Could you check a few things on this model? Use its own coordinates, in mm. A direction names the side the tool comes from. Coordinates: 2 decimals unless noted, no trailing zeros. Loops run counter-clockwise (first coordinate to the right, second up) from the corner with the lowest first, then second, coordinate; pieces in that order, holes last. Notation, with made-up numbers: M 40,84 L 44,84 A30 cw 44,114 Z; hole C -29.75,-31.75 d8. An arc over 180 degrees is marked long. Write each question's results on one line, items separated by ' | '.
```python
from build123d import *

# Parameters (mm, degrees)
F0_R     = 12.5
F0_R_2   = 7
F1_DEPTH = 40
F2_DEPTH = 15


with BuildPart() as f1:
    # F0 (on Top) → F1 (new body)
    with BuildSketch(Plane.XY):
        Circle(F0_R)
        Circle(F0_R_2, mode=Mode.SUBTRACT)
    extrude(amount=F1_DEPTH)

    # F0 (on Top) → F2 (join)
    with BuildSketch(Plane.XY):
        Circle(F0_R_2)
        with BuildLine():
            ThreePointArc((1.658312, 2.5), (2.643382, 1.418637), (3, 0))
            ThreePointArc((3, 0), (-1.418637, -2.643382), (-1.658312, 2.5))
            ThreePointArc((-1.658312, 2.5), (0, 3), (1.658312, 2.5))
        make_face(mode=Mode.SUBTRACT)
        with BuildLine():
            Line((-1.658312, 2.5), (1.658312, 2.5))
            ThreePointArc((1.658312, 2.5), (0, 3), (-1.658312, 2.5))
        make_face()
    extrude(amount=F2_DEPTH)


solid = f1.part
```
(1) Imagine slicing it at C-C, the plane y = 4. List the corners of the cut face in (x, z) for me, and give its area (3 significant figures).
Reported:
outline: M -11.84,0 L 11.84,0 L 11.84,40 L 5.74,40 L 5.74,15 L -5.74,15 L -5.74,40 L -11.84,40 Z | area: 660 mm2
(2) Will these pins go through, and if not, where does the flat tip stop? P1, Ø12, axis at y = -10, z = 15.5, coming from the +X side; P2, Ø1, axis at x = -2, z = 9, coming from the +Y side; P3, Ø12, axis at x = -8, z = 5, coming from the -Y side.
Reported:
P1: stops at x = 11.84 | P2: stops at y = 12.41 | P3: stops at y = -12.34
(3) Imagine slicing it at A-A, the plane x = 0. List the corners of the cut face in (y, z) for me.
Reported:
outline: M -12.5,0 L -3,0 L -3,15 L -7,15 L -7,40 L -12.5,40 Z; M 2.5,0 L 12.5,0 L 12.5,40 L 7,40 L 7,15 L 2.5,15 Z
(4) Imagine slicing it at D-D, the plane x = -5.5. List the corners of the cut face in (y, z) for me, and give its area (3 significant figures).
Reported:
outline: M -11.22,0 L 11.22,0 L 11.22,40 L 4.33,40 L 4.33,15 L -4.33,15 L -4.33,40 L -11.22,40 Z | area: 681 mm2
(5) If we mould it in two halves opening along Y, with no side actions, what happens to faces 3 (the flat face through (0, 2.5, 7)), 4 (the cylindrical face through (11.923, 3.755, 19.72)), 5 (the flat face through (0, 3, 0))? For each: released by +Y, released by -Y, zero draft, split by the parting line, or undercut.
Reported:
face 3: undercut | face 4: split by the parting line | face 5: zero draft
(6) Imagine slicing it at B-B, the plane z = 8.5. List the corners of the cut face in (x, y) for me.
Reported:
outline: C 0,0 d25; hole M -1.66,2.5 A3 ccw long 1.66,2.5 Z
(7) Please list where these lines run through material, in increasing order: probe 1 along Y at (x, z) = (0, 23); probe 2 along Y at (x, z) = (0, 11.25); probe 3 along X at (y, z) = (-3, 34). Write a range as from..to.
Reported:
probe 1: y = -12.5..-7, 7..12.5 | probe 2: y = -12.5..-3, 2.5..12.5 | probe 3: x = -12.13..-6.32, 6.32..12.13
(8) Which directions (+Z, -Z, +X, -X, +Y, -Y) give clear straight access to the entire face, cutting with the end or side of a thin tool? Please do faces 1 (the flat face through (5.4, -5.4, 40)), 2 (the flat face through (1, -3, 15)).
Reported:
face 1: +Z, +X, -X, +Y, -Y | face 2: +Z
